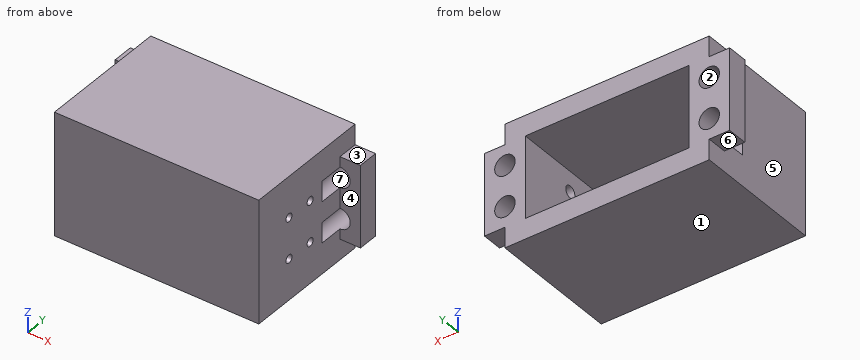
```python
from build123d import *

# Parameters (mm, degrees)
SKETCH1_W           = 50
SKETCH1_H           = 30
SKETCH1_W_2         = 40
SKETCH1_H_2         = 20
BOSS_EXTRUDE1_DEPTH = 26.9
SKETCH2_W           = 10
SKETCH2_H           = 20
SKETCH2_R           = 2.5
BOSS_EXTRUDE2_DEPTH = 5
SKETCH3_R           = 2.5
CUT_EXTRUDE1_DEPTH  = 11
SKETCH5_R           = 1.5
CUT_EXTRUDE3_DEPTH  = 3
SKETCH6_R           = 1
CUT_EXTRUDE4_DEPTH  = 9
SKETCH7_W           = 50
SKETCH7_H           = 30
BOSS_EXTRUDE3_DEPTH = 5


with BuildPart() as part:
    # Sketch1 → Boss-Extrude1 (new body)
    with BuildSketch(Plane(origin=(0, 0, 0), x_dir=(1, 0, 0), z_dir=(0, 1, 0))):
        Rectangle(SKETCH1_W, SKETCH1_H)
        Rectangle(SKETCH1_W_2, SKETCH1_H_2, mode=Mode.SUBTRACT)
    extrude(amount=BOSS_EXTRUDE1_DEPTH)

    # Sketch2 → Boss-Extrude2 (add)
    # profile 1 of 2: a face of its own
    with BuildSketch(Plane(origin=(0, 26.9, 0), x_dir=(1, 0, 0), z_dir=(0, 1, 0))):
        with Locations((25, 0)):
            Rectangle(SKETCH2_W, SKETCH2_H)
        with Locations((25, 5)):
            Circle(SKETCH2_R, mode=Mode.SUBTRACT)
        with Locations((25, -5)):
            Circle(SKETCH2_R, mode=Mode.SUBTRACT)
    # profile 2 of 2: a face of its own
    with BuildSketch(Plane(origin=(0, 26.9, 0), x_dir=(1, 0, 0), z_dir=(0, 1, 0))):
        with Locations((-25, 0)):
            Rectangle(SKETCH2_W, SKETCH2_H)
        with Locations((-25, -5)):
            Circle(SKETCH2_R, mode=Mode.SUBTRACT)
        with Locations((-25, 5)):
            Circle(SKETCH2_R, mode=Mode.SUBTRACT)
    extrude(amount=-BOSS_EXTRUDE2_DEPTH)

    # Sketch3 → Cut-Extrude1 (cut)
    with BuildSketch(Plane(origin=(0, 26.9, 0), x_dir=(1, 0, 0), z_dir=(0, 1, 0))):
        with Locations(Location((-25, 5, 0), (0, 0, 90))):
            Circle(SKETCH3_R)
        with Locations(Location((-25, -5, 0), (0, 0, 90))):
            Circle(SKETCH3_R)
        with Locations(Location((25, -5, 0), (0, 0, 270))):
            Circle(SKETCH3_R)
        with Locations(Location((25, 5, 0), (0, 0, 270))):
            Circle(SKETCH3_R)
    extrude(amount=-CUT_EXTRUDE1_DEPTH, mode=Mode.SUBTRACT)

    # Sketch5 → Cut-Extrude3 (cut)
    with BuildSketch(Plane.ZY.offset(-20)):
        with Locations((-5, 12)):
            Circle(SKETCH5_R)
        with Locations((-5, 5)):
            Circle(SKETCH5_R)
        with Locations((5, 12)):
            Circle(SKETCH5_R)
        with Locations((5, 5)):
            Circle(SKETCH5_R)
    extrude(amount=-CUT_EXTRUDE3_DEPTH, mode=Mode.SUBTRACT)

    # Sketch6 → Cut-Extrude4 (cut)
    with BuildSketch(Plane.ZY.offset(-23)):
        with Locations((-5, 12)):
            Circle(SKETCH6_R)
        with Locations((5, 12)):
            Circle(SKETCH6_R)
        with Locations((-5, 5)):
            Circle(SKETCH6_R)
        with Locations((5, 5)):
            Circle(SKETCH6_R)
    extrude(amount=-CUT_EXTRUDE4_DEPTH, mode=Mode.SUBTRACT)

    # Sketch7 → Boss-Extrude3 (add)
    with BuildSketch(Plane.XZ):
        Rectangle(SKETCH7_W, SKETCH7_H)
    extrude(amount=BOSS_EXTRUDE3_DEPTH)


solid = part.part
```
Input: part model. Units: mm. Frame: model coordinates. Face numbers are marked on the shaded views. A direction names the side the tool comes from. Round coordinates to 2 decimals unless told otherwise and drop trailing zeros. Loops run counter-clockwise (first coordinate to the right, second up) from the corner with the lowest first, then second, coordinate; pieces in that order, holes last. Notation, with made-up numbers: (46, -6) -> (79, -6) arc R20 cw to (79, 17) -> close; hole circle Ø3 at (0, 19). An arc over 180 degrees is marked (long way). One line per item, written item: value.
(1) Mould query, pull axis Z, two halves, no side actions, for the marked faces 5, 6 and 7. Classes: pulls with the +Z half, pulls with the -Z half, needs draft (parallel to the pull), parting line crosses it, or undercut.
Geometry check:
face 5: needs draft
face 6: pulls with the -Z half
face 7: undercut
(2) Set-up query: the marked faces 1, 2, 3 and 4. Return all of +Z, -Z, +X, -X, +Y, -Y with unobstructed straight access to the full face (end or side cutting, diameter ignored); none if empty.
Geometry check:
face 1: -Z, +X, -X, +Y, -Y
face 2: +Y
face 3: +Z, +X, +Y, -Y
face 4: +Z, -Z, +X, -Y
(3) Pin query (flat end, axial travel): pin 1 (2.5 mm diameter, centred on y = 5.5, z = -4.5, fed in from -X); pin 2 (3 mm diameter, centred on y = 9.5, z = -5, fed in from +X); pin 3 (0.8 mm diameter, centred on x = 23, z = 6, fed in from +Y); pin 4 (1.5 mm diameter, centred on x = 5.5, z = 8.5, fed in from +Y). Return the tip coordinate at first contact, or that it passes through.
Geometry check:
pin 1: x = -25
pin 2: x = 25
pin 3: y = 26.9
pin 4: y = 0
(4) Section A-A (y = 12). Return the cut outline in (x, z), plus the area to 3 significant figures.
Geometry check:
outline: (-25, -15) -> (25, -15) -> (25, -6) -> (23, -6) -> (23, -6.5) -> (20, -6.5) -> (20, -10) -> (-20, -10) -> (-20, 10) -> (20, 10) -> (20, 6.5) -> (23, 6.5) -> (23, 6) -> (25, 6) -> (25, 15) -> (-25, 15) -> close; (20, -3.5) -> (23, -3.5) -> (23, -4) -> (25, -4) -> (25, 4) -> (23, 4) -> (23, 3.5) -> (20, 3.5) -> close
area: 674 mm2
(5) Material intervals for line 1 (Y direction, x = 23.6, z = -5); line 2 (Z direction, x = -0.5, y = 1.5); line 3 (X direction, y = 20.5, z = 9), sorted ascending. Write a range as [from, to].
Geometry check:
line 1: [-5, 4], [6, 11], [13, 15.9]
line 2: [-15, -10], [10, 15]
line 3: [-25, -20], [20, 25]
(6) Section B-B (x = 12). Return the cut outline in (y, z).
Geometry check:
outline: (-5, -15) -> (26.9, -15) -> (26.9, -10) -> (0, -10) -> (0, 10) -> (26.9, 10) -> (26.9, 15) -> (-5, 15) -> close
(7) Section C-C (y = 18). Return the cut outline in (x, z), plus the area to 3 significant figures.
Geometry check:
outline: (-25, -15) -> (25, -15) -> (25, -7.5) arc R2.5 cw to (25, -2.5) -> (25, 2.5) arc R2.5 cw to (25, 7.5) -> (25, 15) -> (-25, 15) -> (-25, 7.5) arc R2.5 cw to (-25, 2.5) -> (-25, -2.5) arc R2.5 cw to (-25, -7.5) -> close; hole (-20, -10) -> (20, -10) -> (20, 10) -> (-20, 10) -> close
area: 661 mm2
(8) Section D-D (z = 0). Return the cut outline in (x, y), plus the area to 3 significant figures.
Geometry check:
outline: (-30, 21.9) -> (-25, 21.9) -> (-25, -5) -> (25, -5) -> (25, 21.9) -> (30, 21.9) -> (30, 26.9) -> (20, 26.9) -> (20, 0) -> (-20, 0) -> (-20, 26.9) -> (-30, 26.9) -> close
area: 569 mm2
